Here's how the part is built. I have some questions about the finished solid (model axes, mm). Coordinates: 2 decimals unless noted, no trailing zeros. Write each loop counter-clockwise with the first axis right and the second up, starting at its lowest first coordinate (ties: lowest second). Pieces come first, ordered by that corner, then holes. Notation, with made-up numbers: M 69.5,60.5 L 119.5,60.5 A23 ccw 119.5,69.5 Z; hole C 79,-39 d4. An arc over 180 degrees is marked long. Use one line per item in the form item = value. Start each with the question number.
1. I want a section at D-D, the plane z = 12. List the corners of the cut face in (x, y) for me.
2. I want a section at C-C, the plane x = -62. List the corners of the cut face in (y, z) for me, plus the area to 3 significant figures.
3. Thinking about a two-plate mould opening in X: for faces 1 (the face through (-32.055, -13, 3)), 2 (the face through (-127.304, -13, 3)), 3 (the face through (-45.145, -12.543, 4.222)), 4 (the face through (-80, -13, -34.411)), which applies, released by +X, released by -X, zero draft, split by the parting line, or undercut?
4. I want a section at A-A, the plane z = 26. List the corners of the cut face in (x, y) for me.
5. I want a section at B-B, the plane y = -12.7. List the corners of the cut face in (x, z) for me.
6. Please list where these lines run through material, in increasing order: line 1 along Z through (x, y) = (-79.5, -8.5); line 2 along X through (y, z) = (-11.5, 14); line 3 along X through (y, z) = (-15.75, 31). Write a range as [from, to].
7. I'm going to push a flat-ended pin straight in: pin 1 Ø6.5 at (x, y) = (-117.78, -12.7) entering from +Z. Where does the tip first touch, or does it pass through?
from build123d import *

# Parameters (mm, degrees)
F0_W     = 95.25
F0_H     = 76.2
F1_DEPTH = 25.4
F2_R     = 23.749
F3_DEPTH = 25.4
F4_R     = 3.5687
F5_DEPTH = 76.201


with BuildPart() as f1:
    # F0 (on Front) → F1 (new body)
    with BuildSketch(Plane.XZ):
        with Locations((-79.6795, 3.688855)):
            Rectangle(F0_W, F0_H)
    extrude(amount=F1_DEPTH)

    # F2 (on face) → F3 (cut)
    with BuildSketch(Plane.XZ.offset(25.4)):
        with Locations((-79.6795, 3.688855)):
            Circle(F2_R)
    extrude(amount=-F3_DEPTH, mode=Mode.SUBTRACT)

    # F4 (on face) → F5 (cut, through all)
    with BuildSketch(Plane.XY.offset(41.788855)):
        with Locations((-41.5795, -12.7)):
            Circle(F4_R)
        with Locations((-117.7795, -12.7)):
            Circle(F4_R)
    extrude(amount=-F5_DEPTH, mode=Mode.SUBTRACT)


solid = f1.part
Answer list:
q1.outline = M -127.3,-25.4 L -101.93,-25.4 L -101.93,0 L -127.3,0 Z; M -57.43,-25.4 L -32.05,-25.4 L -32.05,0 L -57.43,0 Z; hole C -117.78,-12.7 d7.14; hole C -41.58,-12.7 d7.14
q2.outline = M -25.4,-34.41 L 0,-34.41 L 0,-12.17 L -25.4,-12.17 Z; M -25.4,19.55 L 0,19.55 L 0,41.79 L -25.4,41.79 Z
q2.area = 1,130 mm²
q3.face_1 = released by +X
q3.face_2 = released by -X
q3.face_3 = undercut
q3.face_4 = zero draft
q4.outline = M -127.3,-25.4 L -87.82,-25.4 L -87.82,0 L -127.3,0 Z; M -71.54,-25.4 L -32.05,-25.4 L -32.05,0 L -71.54,0 Z; hole C -117.78,-12.7 d7.14; hole C -41.58,-12.7 d7.14
q5.outline = M -127.3,-34.41 L -121.35,-34.41 L -121.35,41.79 L -127.3,41.79 Z; M -114.21,-34.41 L -45.15,-34.41 L -45.15,41.79 L -114.21,41.79 Z; M -38.01,-34.41 L -32.05,-34.41 L -32.05,41.79 L -38.01,41.79 Z; hole C -79.68,3.69 d47.5
q6.line_1 = [-34.41, -20.06], [27.44, 41.79]
q6.line_2 = [-127.3, -121.14], [-114.42, -101.07], [-58.29, -44.94], [-38.22, -32.05]
q6.line_3 = [-127.3, -119.63], [-115.93, -43.43], [-39.73, -32.05]
q7.pin_1 = through
